The drawing under review shows one solid part. Ordinate dimensions are in mm from its lowest x, y, z. A direction names the side the tool comes from. Coordinates: 2 decimals unless noted, no trailing zeros. Write each loop counter-clockwise with the first axis right and the second up, starting at its lowest first coordinate (ties: lowest second). Pieces come first, ordered by that corner, then holes.
Q1. Take a section at D-D (z = 75). Give the boundary of the cut face in (x, y), and give its area (3 significant figures).
Q2. Take a section at C-C (x = 56.5). Give the boundary of the cut face in (y, z), and give its area (3 significant figures).
Q3. Mouldability with a two-part tool opening along Y and no side actions: class the marked faces 3, 4, 5 and 6 as pulls with the +Y half, pulls with the -Y half, needs draft (parallel to the pull), parting line crosses it, or undercut.
Q4. For probe 1 along Y at (x, z) = (40.5, 138); probe 2 along X at (y, z) = (29, 55); probe 3 along Z at (x, y) = (63, 41), list the stretches that pass through material, from the lowest coordinate up.
Q5. Machinability: for the marked faces 1 and 2, which of the approach directions +Z, -Z, +X, -X, +Y, -Y give a long, thin tool a straight path to every point of the face, cutting with its end or side? Answer none if there is none.
Q6. Take a section at B-B (y = 5.5). Give the boundary of the cut face in (x, z), and give its area (3 significant figures).
Q7. Insertion check: pin 1 (1.5 mm diameter, centred on x = 114.5, z = 42.5, fed in from -Y); pin 2 (4 mm diameter, centred on x = 92.5, y = 66.5, fed in from -Z); pin 3 (8 mm diameter, centred on x = 60, y = 67, fed in from -Z); pin 4 (2 mm diameter, centred on x = 59, y = 31.5, fed in from +Z). Each pin has a flat end and moves straight along its axis. Give the tip position at first contact, or say it passes through.
Q8. Take a section at A-A (x = 127.5). Give the boundary of the cut face in (y, z), and give its area (3 significant figures).
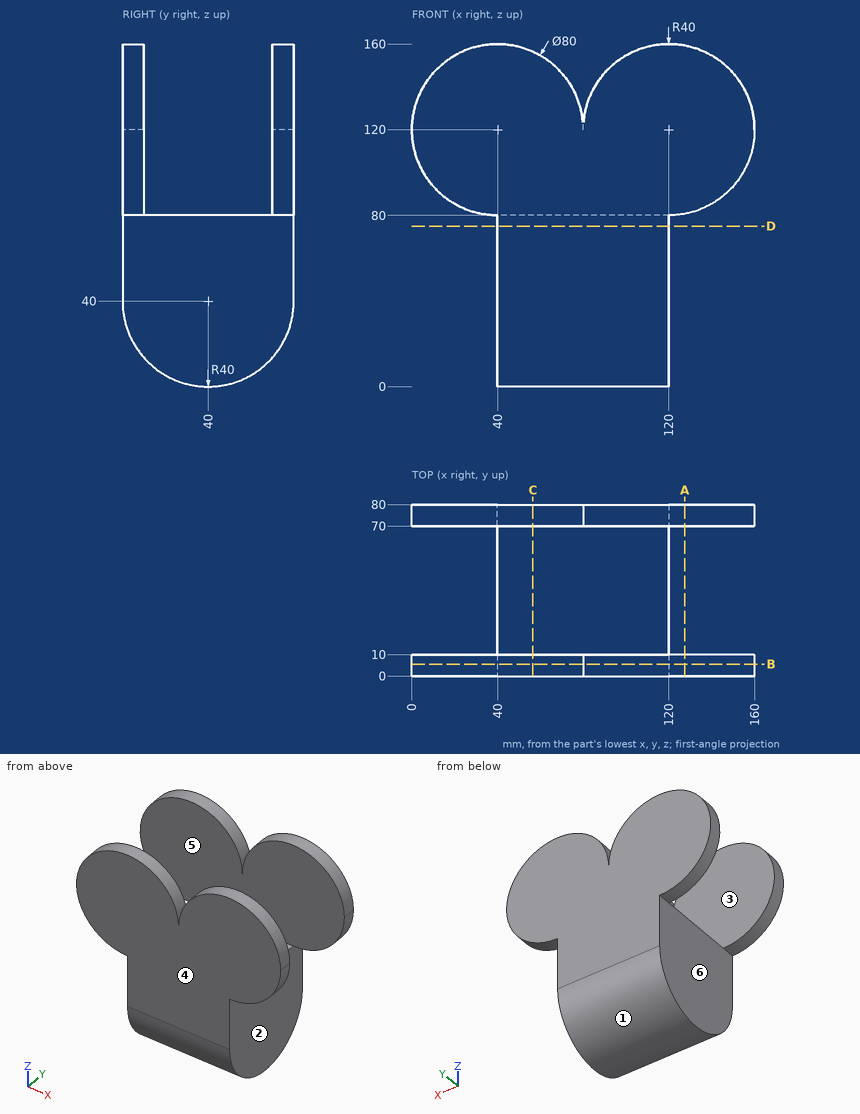
Response:
1. outline: (40, 0) - (120, 0) - (120, 80) - (40, 80) - close
1. area: 6,400 mm2
2. outline: (0, 40) arc R40 ccw to (80, 40) - (80, 156.44) - (70, 156.44) - (70, 80) - (10, 80) - (10, 156.44) - (0, 156.44) - close
2. area: 7,240 mm2
3. face 3: undercut
3. face 4: pulls with the -Y half
3. face 5: undercut
3. face 6: needs draft
4. probe 1: y = 0 to 10, 70 to 80
4. probe 2: x = 40 to 120
4. probe 3: z = 0.01 to 80
5. face 1: -Z, +X, -X
5. face 2: -Z, +X, +Y, -Y
6. outline: (40, 19.76) - (120, 19.76) - (120, 80) arc R40 ccw (long way) to (80, 120) arc R40 ccw (long way) to (40, 80) - close
6. area: 15,600 mm2
7. pin 1: stops at y = 0
7. pin 2: stops at z = 8.38
7. pin 3: stops at z = 7.27
7. pin 4: stops at z = 80
8. outline: (0, 80.71) - (10, 80.71) - (10, 159.29) - (0, 159.29) - close; (70, 80.71) - (80, 80.71) - (80, 159.29) - (70, 159.29) - close
8. area: 1,570 mm2
